Job drawing, mm, ordinate dimensions from the low corner. One solid piece. Give positions to 0.01 mm unless a question says otherwise; leave off trailing zeros. Loops run counter-clockwise (first coordinate to the right, second up) from the corner with the lowest first, then second, coordinate; pieces in that order, holes last. Notation, with made-up numbers: M 20,85 L 29,85 A25 ccw 29,110 Z; hole C 75,44.5 d1. An arc over 180 degrees is marked long. Put each result on its own line as item: value.
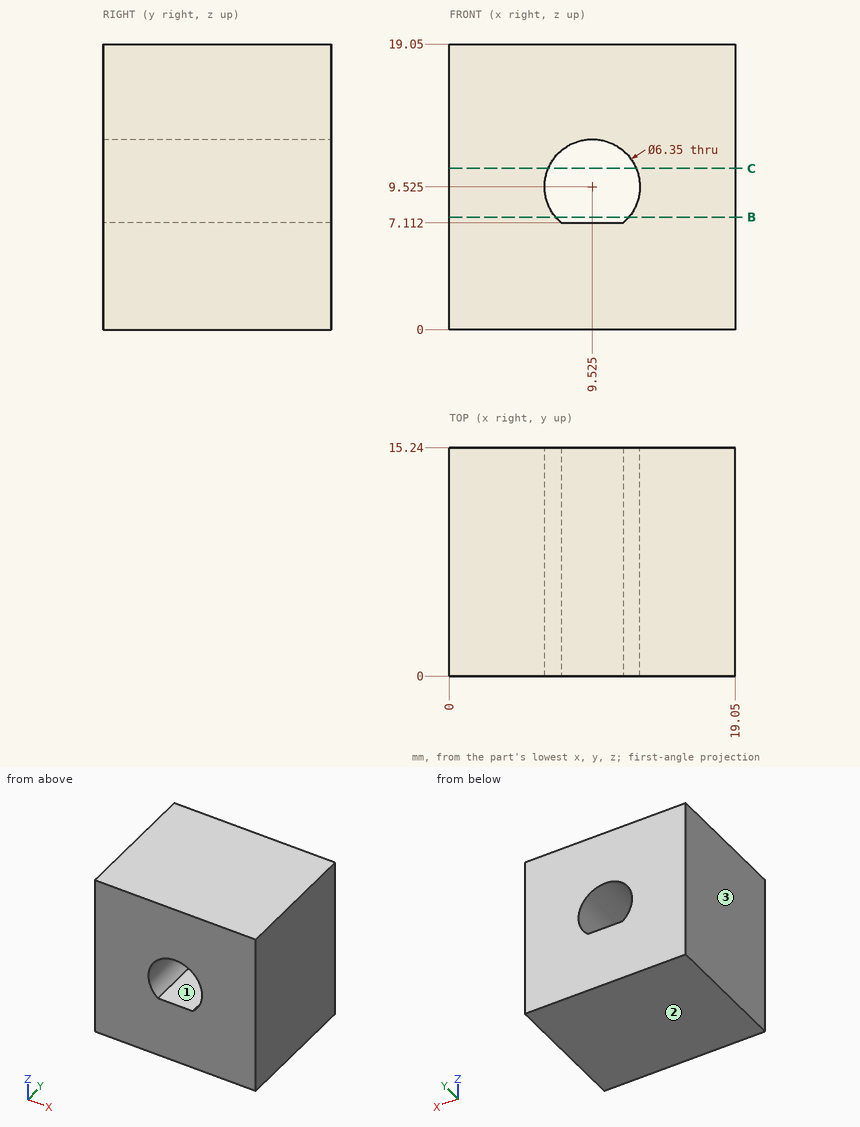
Q1. Probe line 1 (X direction, y = 13.25, z = 9.5); line 2 (X direction, y = 7, z = 8.75); line 3 (Z direction, x = 11.75, y = 11). List the from-to ranges inside material, lowest first. Write a range as from..to.
Here are the results:
line 1: 0..6.35, 12.7..19.05
line 2: 0..6.45, 12.6..19.05
line 3: 0..7.26, 11.79..19.05
Q2. Drop a flat-ended pin along its axis: pin 1 Ø8.5 at (x, z) = (9.525, 9.525) entering from +Y. Give the stop position or say it passes through.
Here are the results:
pin 1: y = 15.24
Q3. Slice it at B-B (z = 7.5). List the corners of the cut face in (x, y).
Here are the results:
outline: M 0,0 L 7.08,0 L 7.08,15.24 L 0,15.24 Z; M 11.97,0 L 19.05,0 L 19.05,15.24 L 11.97,15.24 Z
Q4. Slice it at C-C (z = 10.75). List the corners of the cut face in (x, y).
Here are the results:
outline: M 0,0 L 6.6,0 L 6.6,15.24 L 0,15.24 Z; M 12.45,0 L 19.05,0 L 19.05,15.24 L 12.45,15.24 Z
Q5. Mould opens along X. For the marked faces 1, 2 and 3 say: pulls with the +X half, pulls with the -X half, needs draft (parallel to the pull), parting line crosses it, or undercut.
Here are the results:
face 1: undercut
face 2: needs draft
face 3: pulls with the -X half
